from build123d import *

# Parameters (mm, degrees)
SKETCH2_W           = 22.16775651
SKETCH2_H           = 25.111868119
CUT_EXTRUDE1_DEPTH  = 9
BOSS_EXTRUDE1_DEPTH = 1


with BuildPart() as part:
    # Sketch1 → Revolve1 (revolve)
    with BuildSketch(Plane.XY):
        with BuildLine():
            Line((6.5, 0), (9, 0))
            add(Edge.make_bspline(
                [(0, 20.35), (1.675966842, 20.428176516), (5.66035993, 19.372470149), (8.740520085, 10.941984052), (8.794057121, 4.785623995), (9, 0)],
                knots=[0, 0, 0, 0, 0.209086974, 0.440428739, 1, 1, 1, 1], degree=3))
            Line((0, 20.35), (0, 17.85))
            add(Edge.make_bspline(
                [(0, 17.85), (1.248468613, 18.003104069), (3.434295374, 16.83334968), (6.617297319, 10.514055415), (6.220398856, 4.532307189), (6.5, 0)],
                knots=[0, 0, 0, 0, 0.174730572, 0.328981961, 1, 1, 1, 1], degree=3))
        make_face()
    revolve(axis=Axis((0, 24.080193906, 0), (0, -1, 0)))

    # Sketch2 → Cut-Extrude1 (cut)
    with BuildSketch(Plane.XY.offset(9)):
        with Locations((0.864101602, 11.007607196)):
            Rectangle(SKETCH2_W, SKETCH2_H)
    extrude(amount=-CUT_EXTRUDE1_DEPTH, mode=Mode.SUBTRACT)

    # Sketch3 → Boss-Extrude1 (add)
    with BuildSketch(Plane.XY):
        with BuildLine():
            Line((-7.75, 0), (7.75, 0))
            add(Edge.make_bspline(
                [(-7.75, 0), (-8.003711251, 4.491264664), (-7.661665361, 10.48327828), (-4.662420922, 18.274599737), (0.148702201, 19.617208041), (4.677365419, 17.883192424), (7.773890001, 10.39627401), (7.411285563, 4.341150012), (7.75, 0)],
                knots=[0, 0, 0, 0, 0.289463592, 0.419223785, 0.501869976, 0.592483788, 0.714941347, 1, 1, 1, 1], degree=3))
        make_face()
    extrude(amount=-BOSS_EXTRUDE1_DEPTH)


solid = part.part
For this review, take the finished solid that the model builds, in its own axes (mm). A direction names the side the tool comes from. Round coordinates to 2 decimals unless told otherwise and drop trailing zeros. Use CSV: the item, a comma, the result in double quotes.
(1) For faces 1 (the face through (0, 10, 0)), 2 (the face through (0, 7, -1)), list the 3-axis set-ups (+Z, -Z, +X, -X, +Y, -Y) from which the entire face can be reached by the end or side of a thin tool; tool diameter is ignored.
Computed values:
face 1,"+Z, +X, -X, +Y, -Y"
face 2,"-Y"
(2) Clearance check with flat-ended pins moving along their axes: P1, Ø2, axis at y = 4, z = -6, coming from the -X side; P2, Ø10.5, axis at x = 1, y = 10, coming from the -Z side; P3, Ø8, axis at x = -5.5, y = 16, coming from the -Z side. State where each tip first meets the part, or that it passes through.
Computed values:
P1,"x = -7.28"
P2,"z = -8.79"
P3,"z = -7.21"
(3) To check wall thickness, follow L1, parallel to Z at x = -2.5, y = 15.75; L2, parallel to X at y = 2.5, z = -4; L3, parallel to Z at x = -3, y = 9.5. State the ranges of each line that lie inside material, in increasing order. Write a range as [from, to].
Computed values:
L1,"[-6.42, -2.94], [-1, 0]"
L2,"[-7.95, -4.99], [4.99, 7.95]"
L3,"[-7.81, -5.13], [-1, 0]"
